Answer from the drawing. Dimensions are ordinates in mm from the lowest x, y and z of the part. A direction names the side the tool comes from. Give positions to 0.01 mm unless a question says otherwise; leave off trailing zeros. Loops run counter-clockwise (first coordinate to the right, second up) from the corner with the lowest first, then second, coordinate; pieces in that order, holes last. Notation, with made-up numbers: M 47,45.25 L 58,45.25 A18 cw 58,52.25 Z; hole C 40.25,65.25 d10. An arc over 180 degrees is marked long. Return JSON: item names as keys, results as strings. Group by question number.
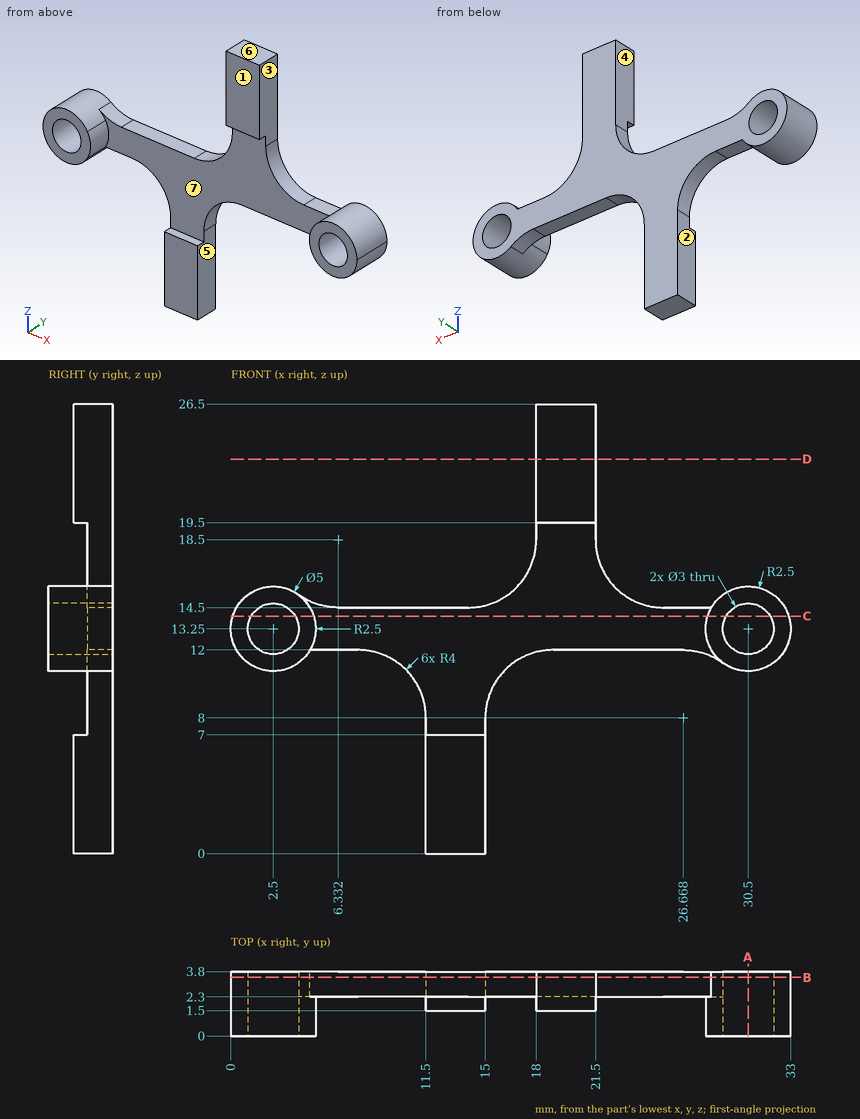
1. Find section A-A (x = 30.5). Write down the section's boundary in (y, z).
2. For the marked faces 1, 2, 3 and 4, determine the directions among +Z, -Z, +X, -X, +Y, -Y from which every point of the face is accessible in a straight line to the end or side of a thin tool.
3. Find section B-B (y = 3.45). State how many separate pieces and enclosed holes the cut face has.
4. Straight lines are drawn through the part: line 1 along X through (y, z) = (1, 13.25); line 2 along X through (y, z) = (2.4, 13.25); line 3 along Z through (x, y) = (2.5, 2.7). For each, find the intervals that lie inside material, in ascending order.
5. Flat-ended cylindrical pins translate along their axes: P1, Ø0.7, axis at y = 2.5, z = 5, coming from the +X side; P2, Ø12, axis at x = 22.5, z = 18, coming from the -Y side; P3, Ø1.6, axis at x = 21.5, y = 3, coming from the -Z side; P4, Ø2.5, axis at x = 30.5, z = 13.25, coming from the -Y side. Find the tip coordinate at first contact, or state that the pin passes through.
6. The mould has two halves that part along X. Classify the marked faces 5, 6 and 7: +X half, -X half, draft (parallel to the pull), parting line (faces both ways), or undercut.
7. Find section C-C (z = 14). Write down the section's boundary in (x, y) (1 decimal).
8. Find section D-D (z = 23.25). Write down the section's boundary in (x, y).
Result:
{
 "1": {"outline": "M 0,10.75 L 3.8,10.75 L 3.8,11.75 L 0,11.75 Z; M 0,14.75 L 3.8,14.75 L 3.8,15.75 L 0,15.75 Z"},
 "2": {"face 1": "+Z, -Z, +X, -X, -Y", "face 2": "-Z, -X, +Y, -Y", "face 3": "+Z, +X, +Y, -Y", "face 4": "+Z, -X, +Y, -Y"},
 "3": {"separate pieces": "1", "enclosed holes": "2"},
 "4": {"line 1": "x = 0 to 1, 4 to 5, 28 to 29, 32 to 33", "line 2": "x = 0 to 1, 4 to 29, 32 to 33", "line 3": "z = 10.75 to 11.75, 14.75 to 15.75"},
 "5": {"P1": "stops at x = 15", "P2": "stops at y = 1.5", "P3": "stops at z = 12", "P4": "passes through"},
 "6": {"face 5": "+X half", "face 6": "draft", "face 7": "undercut"},
 "7": {"outline": "M 0.1,0 L 1.2,0 L 1.2,3.8 L 0.1,3.8 Z; M 3.8,0 L 4.9,0 L 4.9,2.3 L 28.1,2.3 L 28.1,0 L 29.2,0 L 29.2,3.8 L 3.8,3.8 Z; M 31.8,0 L 32.9,0 L 32.9,3.8 L 31.8,3.8 Z"},
 "8": {"outline": "M 18,1.5 L 21.5,1.5 L 21.5,3.8 L 18,3.8 Z"}
}
